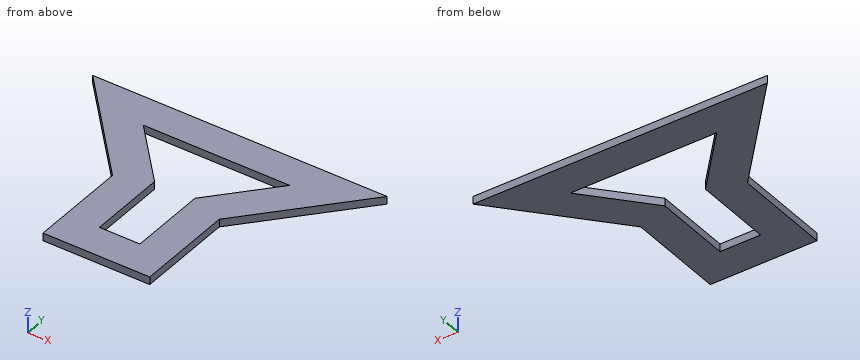
```python
from build123d import *

# Parameters (mm, degrees)
EXTRUDE_2_DEPTH = 10


with BuildPart() as part:
    # Эскиз5 → Бобышка-Вытянуть2 (new body)
    with BuildSketch(Plane.XY):
        Polygon((69.270264014, 2.532805315), (69.270264014, -125.60178411), (-69.270264014, -125.60178411), (-69.270264014, 2.532805315), (-190.995381487, 138.884340659), (190.995381487, 138.884340659), align=None)
        Polygon((-26.270264014, -82.60178411), (26.270264014, -82.60178411), (26.270264014, 18.934099876), (94.96605886, 95.884340659), (-94.96605886, 95.884340659), (-26.270264014, 18.934099876), align=None, mode=Mode.SUBTRACT)
    extrude(amount=EXTRUDE_2_DEPTH)


solid = part.part
```
Design review of the part built by this model. Coordinates are the model's own, in mm. Give positions to 0.01 mm unless a question says otherwise; leave off trailing zeros. Order: outer loops, then holes, each group sorted by start corner. A loop starts at its lowest first (then second) coordinate and runs counter-clockwise, first axis right, second up. Notation, with made-up numbers: M 24,63 L 52,63 A27 cw 52,80 Z; hole C -38.75,54.5 d1. An arc over 180 degrees is marked long. One line per question, with ' | ' between items. Start each with the question number.
Q1. We need section D-D (x = 167.5). Write out the cut boundary in (y, z), plus the area to 3 significant figures.
Q2. We need section A-A (y = -73.5). Write out the cut boundary in (x, z).
Q3. For pin 1 Ø3 at (y, z) = (-69, 5) entering from +X; pin 2 Ø6 at (y, z) = (67, 5) entering from -X; pin 3 Ø5 at (y, z) = (-0.5, 3) entering from -X, all flat-tipped, find the tip position at first contact; note any pin that passes through.
Q4. We need section B-B (x = 15). Write out the cut boundary in (y, z), plus the area to 3 significant figures.
Q5. For L1, parallel to X at y = -51.5, z = 4.25; L2, parallel to Y at x = 1, z = 1; L3, parallel to Y at x = 26.5, z = 6.25, list the stretches that pass through material, from the lowest coordinate up. Write a range as [from, to].
Q6. We need section C-C (z = 6.5). Write out the cut boundary in (x, y).
Returned:
1) outline: M 112.57,0 L 138.88,0 L 138.88,10 L 112.57,10 Z | area: 263 mm2
2) outline: M -69.27,0 L -26.27,0 L -26.27,10 L -69.27,10 Z; M 26.27,0 L 69.27,0 L 69.27,10 L 26.27,10 Z
3) pin 1: x = 69.27 | pin 2: x = -129.5 | pin 3: x = -69.27
4) outline: M -125.6,0 L -82.6,0 L -82.6,10 L -125.6,10 Z; M 95.88,0 L 138.88,0 L 138.88,10 L 95.88,10 Z | area: 860 mm2
5) L1: [-69.27, -26.27], [26.27, 69.27] | L2: [-125.6, -82.6], [95.88, 138.88] | L3: [-125.6, 19.19], [95.88, 138.88]
6) outline: M -191,138.88 L -69.27,2.53 L -69.27,-125.6 L 69.27,-125.6 L 69.27,2.53 L 191,138.88 Z; hole M -94.97,95.88 L -26.27,18.93 L -26.27,-82.6 L 26.27,-82.6 L 26.27,18.93 L 94.97,95.88 Z
